from build123d import *

# Parameters (mm, degrees)
SKETCH1_R               = 12.7
SKETCH1_R_2             = 10.75
BOSS_EXTRUDE1_DEPTH     = 510
CUT_EXTRUDE1_DEPTH      = 510
CUT_EXTRUDE2_DEPTH      = 16
CUT_EXTRUDE2_DEPTH_BACK = 19
SKETCH3_W               = 18.830602732
SKETCH3_H               = 12
SKETCH3_W_2             = 16.984597957
SKETCH5_W               = 9.256693762
SKETCH5_H               = 14.558945698
BOSS_EXTRUDE2_DEPTH     = 10
FILLET1_R               = 3


with BuildPart() as part:
    # Sketch1 → Boss-Extrude1 (new body)
    with BuildSketch(Plane(origin=(0, 0, 0), x_dir=(1, 0, 0), z_dir=(0, 1, 0))):
        with Locations(Location((0, 0, 0), (0, 0, 270))):
            Circle(SKETCH1_R)
        with Locations(Location((0, 0, 0), (0, 0, 270))):
            Circle(SKETCH1_R_2, mode=Mode.SUBTRACT)
    extrude(amount=BOSS_EXTRUDE1_DEPTH)

    # Sketch2 → Cut-Extrude1 (cut)
    with BuildSketch(Plane(origin=(0, 510, 0), x_dir=(1, 0, 0), z_dir=(0, 1, 0))):
        Polygon((10.406693762, 24.487366984), (10.406693762, -11.087366984), (10.406693762, -15.222442653), (-10.406693762, -15.222442653), (-10.406693762, -10.249436946), (-10.406693762, 23.649436946), align=None)
    extrude(amount=-CUT_EXTRUDE1_DEPTH, mode=Mode.SUBTRACT)


with BuildPart() as cut_extrude1_piece_1:
    # of the separate pieces the step leaves, piece 1, a body of its own (cut_extrude1_pieces)
    add(part.part.solids().sort_by_distance((10.406693762, 0, 7.279472849))[0])


with BuildPart() as cut_extrude1_piece_2:
    # of the separate pieces the step leaves, piece 2, a body of its own (cut_extrude1_pieces)
    add(part.part.solids().sort_by_distance((-10.406693762, 0, -7.279472849))[0])


with BuildPart() as cut_extrude2_tool:
    # Sketch3 → Cut-Extrude2 (new, two sides: drawn at the far end of the back side and taken through both)
    with BuildSketch(Plane(origin=(0, 0, 0), x_dir=(0, 0, -1), z_dir=(1, 0, 0)).offset(-CUT_EXTRUDE2_DEPTH_BACK)):
        with Locations((2.135828517, 6)):
            Rectangle(SKETCH3_W, SKETCH3_H)
        with Locations((1.21282613, 504)):
            Rectangle(SKETCH3_W_2, SKETCH3_H)
    extrude(amount=CUT_EXTRUDE2_DEPTH + CUT_EXTRUDE2_DEPTH_BACK)


with BuildPart() as cut_extrude1_piece_1_1:
    add(cut_extrude1_piece_1.part)

    # Cut-Extrude2: cut by cut_extrude2_tool
    add(cut_extrude2_tool.part, mode=Mode.SUBTRACT)



with BuildPart() as cut_extrude1_piece_2_1:
    add(cut_extrude1_piece_2.part)

    # Cut-Extrude2: cut by cut_extrude2_tool
    add(cut_extrude2_tool.part, mode=Mode.SUBTRACT)


with BuildPart() as cut_extrude1_piece_1_2:
    add(cut_extrude1_piece_1_1.part)

    add(cut_extrude1_piece_2_1.part)  # Boss-Extrude2 merges Cut-Extrude1 piece 2
    # Sketch5 → Boss-Extrude2 (add)
    with BuildSketch(Plane(origin=(0, 355, 0), x_dir=(1, 0, 0), z_dir=(0, 1, 0))):
        with BuildLine():
            Line((12.7, 9.720527151), (-12.7, 9.720527151))
            ThreePointArc((-12.7, 9.720527151), (-15.678586565, 0.070527151), (-12.7, -9.579472849))
            Line((-12.7, -9.579472849), (12.7, -9.579472849))
            ThreePointArc((12.7, -9.579472849), (15.616851042, 0.070527151), (12.7, 9.720527151))
        make_face()
        with Locations((-5.778346881, 0)):
            Rectangle(SKETCH5_W, SKETCH5_H, mode=Mode.SUBTRACT)
        with Locations((5.778346881, 0)):
            Rectangle(SKETCH5_W, SKETCH5_H, mode=Mode.SUBTRACT)
    boss_extrude2 = extrude(amount=BOSS_EXTRUDE2_DEPTH)

    # Fillet1
    fillet1_edges = [cut_extrude1_piece_1_2.edges().sort_by_distance(p)[0] for p in [
        (-12.7, 360, -9.720527151),
        (-12.7, 360, 9.579472849),
        (12.7, 360, 9.579472849),
        (12.7, 360, -9.720527151),
    ]]
    fillet(fillet1_edges, radius=FILLET1_R)

    # Mirror1: Boss-Extrude2 across plane
    add(boss_extrude2.mirror(Plane.ZX.offset(260)))


solid = cut_extrude1_piece_1_2.part
The model under review builds one solid part; all positions refer to its coordinate system, in mm. A direction names the side the tool comes from. Round coordinates to 2 decimals unless told otherwise and drop trailing zeros. Write each loop counter-clockwise with the first axis right and the second up, starting at its lowest first coordinate (ties: lowest second). Pieces come first, ordered by that corner, then holes. Notation, with made-up numbers: M 29,85 L 62,85 A24 cw 62,117 Z; hole C 72.5,79 d10. An arc over 180 degrees is marked long. Answer as CSV lines item,"result". Start each with the question number.
Q1. Clearance check with flat-ended pins moving along their axes: P1, Ø9.5, axis at x = 0.5, z = -1, coming from the +Y side; P2, Ø4.5, axis at y = 228, z = -3, coming from the -X side; P3, Ø4, axis at y = 384.5, z = 5.5, coming from the +X side; P4, Ø4, axis at x = -7.5, y = 67.5, coming from the -Z side. State where each tip first meets the part, or that it passes through.
Q2. Consider section B-B, the plane x = 6.5. Give the boundary of the cut face in (y, z), then the cut area to 3 significant figures.
Q3. Wall thickness on line 1 along Y through (x, z) = (-8, 8.5); line 2 along X through (y, z) = (226.5, -1.5); line 3 along X through (y, z) = (187.5, 4.5): over which ranges is each line inside the solid? List them lowest first.
Q4. The part is to be moulded in two halves that separate along X. For faces 1 (the face through (-1.15, 160, 0)), 2 (the face through (0, 160, -9.721)), 3 (the face through (15.616, 160.07, 0.073)), say which applies: +X half, -X half, draft (parallel to the pull), parting line (faces both ways), or undercut.
Q5. Tool access review of faces 4 (the face through (12.7, 430.6, 0.1)), 5 (the face through (-15.68, 359.93, -0.19)), 6 (the face through (12.7, 258.7, 0.1)), 7 (the face through (6, 160, 7.279)), 8 (the face through (12.7, 82.5, 0.1)): name each direction out of +Z, -Z, +X, -X, +Y, -Y from which nothing blocks a thin tool from reaching the whole face with its end or side.
Q6. Consider section A-A, the plane y = 443. Give the boundary of the cut face in (x, z).
Result set:
1,P1,"stops at y = 365"
1,P2,"stops at x = -12.68"
1,P3,"stops at x = 12.21"
1,P4,"passes through"
2,outline,"M 155,-9.72 L 165,-9.72 L 165,-7.28 L 155,-7.28 Z; M 155,7.28 L 165,7.28 L 165,9.58 L 155,9.58 Z; M 355,-9.72 L 365,-9.72 L 365,-7.28 L 355,-7.28 Z; M 355,7.28 L 365,7.28 L 365,9.58 L 355,9.58 Z"
2,area,"94.8 mm²"
3,line 1,"y = 155 to 165, 355 to 365"
3,line 2,"x = -12.61 to -10.64, 10.64 to 12.61"
3,line 3,"x = -11.88 to -10.41, 10.41 to 11.88"
4,face 1,"undercut"
4,face 2,"draft"
4,face 3,"+X half"
5,face 4,"+X, +Y"
5,face 5,"-X, +Y, -Y"
5,face 6,"+X"
5,face 7,"+Y, -Y"
5,face 8,"+X, -Y"
6,outline,"M -10.41,-7.28 L -10.41,-2.7 A10.75 cw -10.41,2.7 L -10.41,7.28 A12.7 ccw Z; M 10.41,-7.28 A12.7 ccw 10.41,7.28 L 10.41,2.7 A10.75 cw 10.41,-2.7 Z"
